```python
from build123d import *

# Parameters (mm, degrees)
SUNGU_KIRI_R        = 1
BOSS_EXTRUDE1_DEPTH = 10
SKETCH9_R           = 7.5
CUT_EXTRUDE5_DEPTH  = 5


with BuildPart() as part:
    # sungu kiri → Boss-Extrude1 (new body)
    with BuildSketch(Plane(origin=(0, 0, 0), x_dir=(1, 0, 0), z_dir=(0, 1, 0))):
        with BuildLine():
            Line((-20.214241335, 18.58200887), (-17.903708636, 25.676772527))
            Line((-17.903708636, 25.676772527), (-20.879327355, 22.419581076))
            Line((-20.879327355, 22.419581076), (-23.726014444, 13.678492013))
            ThreePointArc((-23.726014444, 13.678492013), (-25.061399851, 10.98195956), (-26.444409257, 8.309539974))
            ThreePointArc((-26.444409257, 8.309539974), (-27.383764934, 5.63006722), (-27.936945566, 2.845115782))
            ThreePointArc((-27.936945566, 2.845115782), (-28.068014235, 0.18049064), (-27.936945566, -2.484134502))
            ThreePointArc((-27.936945566, -2.484134502), (-27.425713247, -6.715299694), (-26.444409257, -10.862727794))
            ThreePointArc((-26.444409257, -10.862727794), (-25.296755437, -14.61403578), (-23.488374839, -18.095297119))
            ThreePointArc((-23.488374839, -18.095297119), (-22.238356067, -20.131176806), (-20.758136978, -22.006357992))
            ThreePointArc((-20.758136978, -22.006357992), (-13.175246696, -36.755405871), (-4.582277955, -22.571064976))
            ThreePointArc((-4.582277955, -22.571064976), (-4.460378612, -22.299351604), (-4.344569641, -22.024987085))
            ThreePointArc((-4.344569641, -22.024987085), (-4.340995805, -22.01171692), (-4.3373846, -21.998456875))
            ThreePointArc((-4.3373846, -21.998456875), (-4.667057778, -21.129677391), (-5.155481579, -20.33916845))
            ThreePointArc((-5.155481579, -20.33916845), (-7.110923153, -19.117606911), (-9.361873626, -18.618421268))
            ThreePointArc((-9.361873626, -18.618421268), (-11.285784226, -18.376920372), (-13.150188878, -17.844238508))
            ThreePointArc((-13.150188878, -17.844238508), (-15.818147575, -16.60648921), (-18.010368345, -14.645827324))
            ThreePointArc((-18.010368345, -14.645827324), (-20.650416196, -11.005311906), (-22.72256926, -7.01414831))
            ThreePointArc((-22.72256926, -7.01414831), (-21.584958488, 10.98418111), (-6.423603233, 20.74980075))
            Line((-6.423603233, 20.74980075), (-7.667855794, 21.470443038))
            Line((-7.667855794, 21.470443038), (-16.17291449, 19.521519125))
            Line((-16.17291449, 19.521519125), (-20.214241335, 16.223172594))
            Line((-20.214241335, 16.223172594), (-20.214241335, 18.58200887))
        make_face()
        with Locations(Location((-12.843799059, -27.261189607, 0), (0, 0, 270))):
            Circle(SUNGU_KIRI_R, mode=Mode.SUBTRACT)
    extrude(amount=BOSS_EXTRUDE1_DEPTH)

    # Sketch9 → Cut-Extrude5 (cut)
    with BuildSketch(Plane(origin=(0, 10, 0), x_dir=(1, 0, 0), z_dir=(0, 1, 0))):
        with Locations(Location((-12.843799059, -27.261189607, 0), (0, 0, 270))):
            Circle(SKETCH9_R)
    extrude(amount=-CUT_EXTRUDE5_DEPTH, mode=Mode.SUBTRACT)


solid = part.part
```
CAD build for the part. Positions are in the model's coordinates, mm. A direction names the side the tool comes from. Give positions to 0.01 mm unless a question says otherwise; leave off trailing zeros. Order: outer loops, then holes, each group sorted by start corner. A loop starts at its lowest first (then second) coordinate and runs counter-clockwise, first axis right, second up.
(1) Saw through at D-D, the plane z = 4. Give the cut face in (x, y).
(2) Flat gauge pins, fed straight in: pin 1 (4 mm diameter, centred on y = 8.5, z = 3.5, fed in from -X); pin 2 (5 mm diameter, centred on y = 7.5, z = -11.5, fed in from +X); pin 3 (3 mm diameter, centred on y = 7, z = 6.5, fed in from +X). Where does each tip first touch, or does it go through?
(3) Tool access for faces 1 (the flat face through (-18, 0, 17)), 2 (the flat face through (-18.165, 4.93, -17.895)), 3 (the cylindrical face through (-6.52, 7.54, 31.29)), 4 (the cylindrical face through (-11.259, 4.93, 18.382)), 5 (the cylindrical face through (-22.26, 4.93, 20.1)): list every direction of +Z, -Z, +X, -X, +Y, -Y with a clear straight run to the whole face (end or side of a thin tool).
(4) Drill centre lines: L1, parallel to Z at x = -12.5, y = 7.5; L2, parallel to Z at x = -16.75, y = 8.5; L3, parallel to Y at x = -13.25, z = 26. Where is each one in solid material? Low to high.
(5) Saw through at A-A, the plane x = -19. Give the cut face in (y, z).
(6) Saw through at B-B, the plane z = 27.5. Give the cut face in (x, y), then the cut area to 3 significant figures.
(7) Mould opens along X. For faces 6 (the cylindrical face through (-13.46, 4.93, 36.74)), 7 (the flat face through (-11.9, 4.9, -20.5)), 8 (the cylindrical face through (-7.08, 4.93, 19.13)) say: released by +X, released by -X, zero draft, split by the parting line, or undercut.
Results found:
1. outline: (-27.81, 0) - (-23.74, 0) - (-23.74, 10) - (-27.81, 10) - close
2. pin 1: stops at x = -28.02
2. pin 2: stops at x = -19.41
2. pin 3: stops at x = -22.28
3. face 1: +Z, -Z, +X, -X, -Y
3. face 2: +Y, -Y
3. face 3: +Y
3. face 4: +X, +Y, -Y
3. face 5: -X, +Y, -Y
4. L1: z = -20.36 to -19.12, 18.07 to 19.77, 34.75 to 36.75
4. L2: z = -19.05 to -16.54, 15.91 to 20.86, 33.66 to 35.92
4. L3: y = 0 to 5
5. outline: (0, -24.48) - (10, -24.48) - (10, -22.31) - (0, -22.31) - close; (0, -17.21) - (10, -17.21) - (10, -14.46) - (0, -14.46) - close; (0, 13.41) - (10, 13.41) - (10, 22.98) - (5, 22.98) - (5, 31.55) - (10, 31.55) - (10, 34.5) - (0, 34.5) - close
6. outline: (-22.34, 0) - (-13.81, 0) - (-13.81, 5) - (-20.34, 5) - (-20.34, 10) - (-22.34, 10) - close; (-11.87, 0) - (-3.35, 0) - (-3.35, 10) - (-5.35, 10) - (-5.35, 5) - (-11.87, 5) - close
6. area: 105 mm2
7. face 6: split by the parting line
7. face 7: undercut
7. face 8: released by +X
